```python
from build123d import *

# Parameters (mm, degrees)
EXTRUDE_1_DEPTH     = 10
SKETCH_4_R          = 2
CUT_EXTRUDE_1_DEPTH = 13.247448714


with BuildPart() as part:
    # 草图1 → 凸台-拉伸1 (new body)
    with BuildSketch(Plane.XY):
        Polygon((-2.9, 0), (2.9, 0), (2.9, 1.5), (5, 1.5), (5, 2.9), (2.9, 5), (-2.9, 5), (-5, 2.9), (-5, 1.5), (-2.9, 1.5), align=None)
    extrude(amount=-EXTRUDE_1_DEPTH)

    # 草图4 → 切除-拉伸1 (cut, through all)
    with BuildSketch(Plane(origin=(0, 5, 0), x_dir=(1, 0, 0), z_dir=(0, 1, 0))):
        with Locations(Location((0, 5, 0), (0, 0, 270))):
            Circle(SKETCH_4_R)
    extrude(amount=-CUT_EXTRUDE_1_DEPTH, mode=Mode.SUBTRACT)


solid = part.part
```
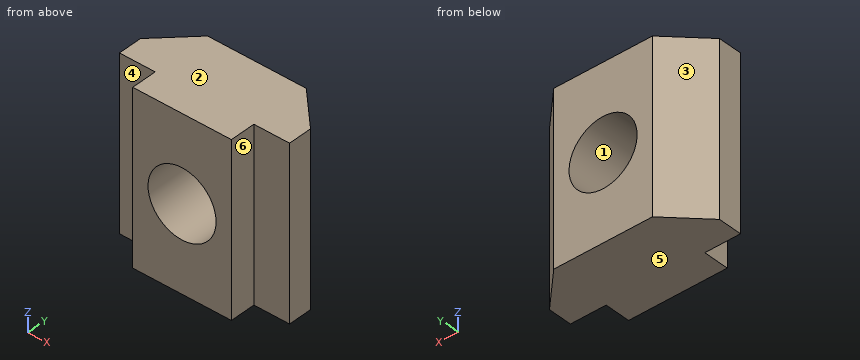
Geometry check sheet. Reference: the model listing, model coordinates, mm. Face numbers are marked on the shaded views. A direction names the side the tool comes from. Round coordinates to 2 decimals unless told otherwise and drop trailing zeros. Order: outer loops, then holes, each group sorted by start corner. A loop starts at its lowest first (then second) coordinate and runs counter-clockwise, first axis right, second up. Notation, with made-up numbers: (53, 55) - (81, 55) arc R17 cw to (81, 72) - close; hole circle Ø9 at (47, 54). An arc over 180 degrees is marked (long way). Use a Markdown table: item, result. Add a question column.
1) Section check D-D (z = -8.5). Record the cut outline in (x, y).
2) Section check A-A (x = 0). Record the cut outline in (y, z), then the cut area to 3 significant figures.
3) Set-up check for the marked faces 4, 5 and 6: record each of +Z, -Z, +X, -X, +Y, -Y from which the full face is reachable in a straight line by a thin tool's end or side.
4) Gauge pin test, flat ends, axial feed: P1, Ø0.6, axis at x = -4, z = -5, coming from the -Y side; P2, Ø1.6, axis at y = 0.5, z = -7, coming from the -X side. Record the tip position at first contact, or that the pin passes through.
5) Section check C-C (z = -4.5). Record the cut outline in (x, y), then the cut area to 3 significant figures.
6) Thickness scan on line 1 along X through (y, z) = (1.6, -5); line 2 along X through (y, z) = (1.25, -5); line 3 along Z through (x, y) = (0.5, 0.35). Record the ranges inside material, lowest first.
7) Mould release check, pull along X, two halves, no side actions. Record for the marked faces 1, 2 and 3: released by +X, released by -X, zero draft, split by the parting line, or undercut.
8) Section check B-B (y = 3.85). Record the cut outline in (x, z), then the cut area to 3 significant figures.
Established:
| question | item | result |
|---|---|---|
| 1 | outline | (-5, 1.5) - (-2.9, 1.5) - (-2.9, 0) - (2.9, 0) - (2.9, 1.5) - (5, 1.5) - (5, 2.9) - (2.9, 5) - (-2.9, 5) - (-5, 2.9) - close |
| 2 | outline | (0, -10) - (5, -10) - (5, -7) - (0, -7) - close; (0, -3) - (5, -3) - (5, 0) - (0, 0) - close |
| 2 | area | 30.0 mm2 |
| 3 | face 4 | +Z, -Z, -X, -Y |
| 3 | face 5 | -Z, +X, -X, +Y, -Y |
| 3 | face 6 | +Z, -Z, +X, -Y |
| 4 | P1 | y = 1.5 |
| 4 | P2 | x = -2.9 |
| 5 | outline | (-5, 1.5) - (-2.9, 1.5) - (-2.9, 0) - (-1.94, 0) - (-1.94, 5) - (-2.9, 5) - (-5, 2.9) - close; (1.94, 0) - (2.9, 0) - (2.9, 1.5) - (5, 1.5) - (5, 2.9) - (2.9, 5) - (1.94, 5) - close |
| 5 | area | 19.9 mm2 |
| 6 | line 1 | -5 to -2, 2 to 5 |
| 6 | line 2 | -2.9 to -2, 2 to 2.9 |
| 6 | line 3 | -10 to -6.94, -3.06 to 0 |
| 7 | face 1 | undercut |
| 7 | face 2 | zero draft |
| 7 | face 3 | released by -X |
| 8 | outline | (-4.05, -10) - (4.05, -10) - (4.05, 0) - (-4.05, 0) - close; hole circle Ø4 at (0, -5) |
| 8 | area | 68.4 mm2 |
